Input: part model. Units: mm. Frame: model coordinates. A direction names the side the tool comes from. Coordinates: 2 decimals unless noted, no trailing zeros. Loops run counter-clockwise (first coordinate to the right, second up) from the corner with the lowest first, then second, coordinate; pieces in that order, holes last. Notation, with made-up numbers: M 73.5,10 L 102.5,10 A19 ccw 102.5,30 Z; hole C 89,-2 d4. An arc over 180 degrees is marked long. Use a Markdown table: item, result. Add a question column.
1. Draft query along Y for faces 1 (the flat face through (-210, -5, 141)), 2 (the flat face through (-198, -179, 147)), 3 (the flat face through (-3, 360, 141)), 4 (the flat face through (-3, -360, 141)). Return one class per face: +Y half, -Y half, draft (parallel to the pull), parting line (faces both ways), or undercut.
2. Line query: L1, parallel to Y at x = -102, z = 58.5; L2, parallel to X at y = 325, z = 117.5; L3, parallel to Z at x = -121, y = 67.5. Output: solid intervals per line, ascending. Write a range as [from, to].
3. Set-up query: faces 5 (the flat face through (-3, -175, 12)), 6 (the flat face through (-3, 5, 0)). Return all of +Z, -Z, +X, -X, +Y, -Y with unobstructed straight access to the full face (end or side cutting, diameter ignored); none if empty.
4. Section C-C on x = 138.5. Output: boundary loops of the cut face in (y, z), then the cut area to 3 significant figures.
5. Pin query (flat end, axial travel): pin 1 (3 mm diameter, centred on x = 136, y = 71.5, fed in from +Z); pin 2 (4 mm diameter, centred on x = -77.5, y = 64, fed in from -Z). Return the tip coordinate at first contact, or that it passes through.
6. Section B-B on z = 110.5. Output: boundary loops of the cut face in (x, y), then the cut area to 3 significant figures.
7. Section A-A on y = 280.5. Output: boundary loops of the cut face in (x, z).
```python
from build123d import *

# Parameters (mm, degrees)
SKETCH_1_W      = 420
SKETCH_1_H      = 720
EXTRUDE_1_DEPTH = 12
SKETCH_2_W      = 420
SKETCH_2_H      = 720
SKETCH_2_W_2    = 396
SKETCH_2_H_2    = 342
EXTRUDE_2_DEPTH = 273


with BuildPart() as part:
    # ｽｹｯﾁ1 → ﾎﾞｽ - 押し出し1 (new body)
    with BuildSketch(Plane.XY):
        Rectangle(SKETCH_1_W, SKETCH_1_H)
    extrude(amount=EXTRUDE_1_DEPTH)

    # ｽｹｯﾁ2 → ﾎﾞｽ - 押し出し2 (add)
    with BuildSketch(Plane.XY.offset(12)):
        Rectangle(SKETCH_2_W, SKETCH_2_H)
        with Locations((0, 177)):
            Rectangle(SKETCH_2_W_2, SKETCH_2_H_2, mode=Mode.SUBTRACT)
        with Locations((0, -177)):
            Rectangle(SKETCH_2_W_2, SKETCH_2_H_2, mode=Mode.SUBTRACT)
    extrude(amount=EXTRUDE_2_DEPTH)


solid = part.part
```
Answers below:
| question | item | result |
|---|---|---|
| 1 | face 1 | draft |
| 1 | face 2 | undercut |
| 1 | face 3 | +Y half |
| 1 | face 4 | -Y half |
| 2 | L1 | y = [-360, -348], [-6, 6], [348, 360] |
| 2 | L2 | x = [-210, -198], [198, 210] |
| 2 | L3 | z = [0, 12] |
| 3 | face 5 | +Z |
| 3 | face 6 | -Z, +X, -X, +Y, -Y |
| 4 | outline | M -360,0 L 360,0 L 360,285 L 348,285 L 348,12 L 6,12 L 6,285 L -6,285 L -6,12 L -348,12 L -348,285 L -360,285 Z |
| 4 | area | 18,500 mm² |
| 5 | pin 1 | stops at z = 12 |
| 5 | pin 2 | stops at z = 0 |
| 6 | outline | M -210,-360 L 210,-360 L 210,360 L -210,360 Z; hole M -198,-348 L 198,-348 L 198,-6 L -198,-6 Z; hole M -198,6 L 198,6 L 198,348 L -198,348 Z |
| 6 | area | 31,500 mm² |
| 7 | outline | M -210,0 L 210,0 L 210,285 L 198,285 L 198,12 L -198,12 L -198,285 L -210,285 Z |
